from build123d import *

# Parameters (mm, degrees)
F1_DEPTH  = 6.35
F3_W      = 31.75
F3_H      = 6.35
F4_DEPTH  = 82.55
F6_DEPTH  = 6.35
F9_W      = 3.175
F9_H      = 12.7
F10_DEPTH = 222.25


with BuildPart() as f1:
    # F0 (on Front) → F1 (new body)
    with BuildSketch(Plane.XZ):
        Polygon((-41.275, 64.447084), (-41.275, 104.775), (-111.125, 104.775), align=None)
        Polygon((0, 104.775), (-41.275, 104.775), (-41.275, 64.447084), (-41.275, -53.975), (0, -53.975), align=None)
    extrude(amount=-F1_DEPTH)

    # F2: F1 across plane


with BuildPart() as f1_1:
    add(f1.part)
    add(f1.part.mirror(Plane.YZ))

    # F3 (on Front) → F4 (join)
    with BuildSketch(Plane.XZ):
        with Locations((0, -50.8)):
            Rectangle(F3_W, F3_H)
    extrude(amount=F4_DEPTH)

    # F5 (on face) → F6 (join)
    with BuildSketch(Plane.YZ.offset(15.875)):
        Polygon((0, -22.225), (-25.4, -47.625), (0, -47.625), align=None)
    extrude(amount=-F6_DEPTH)

    # F7: F1 across plane


with BuildPart() as f1_2:
    add(f1_1.part)
    add(f1_1.part.mirror(Plane.YZ))

    # F9 (on offset) → F10 (cut)
    with BuildSketch(Plane.YZ.offset(111.125)):
        with Locations((1.5875, 98.425)):
            Rectangle(F9_W, F9_H)
    extrude(amount=-F10_DEPTH, mode=Mode.SUBTRACT)


solid = f1_2.part
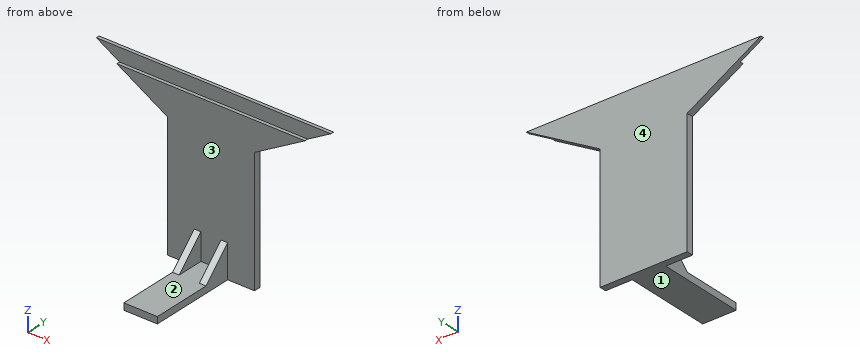
Geometry check sheet. Reference: the model listing, model coordinates, mm. Face numbers are marked on the shaded views. A direction names the side the tool comes from. Round coordinates to 2 decimals unless told otherwise and drop trailing zeros. Write each loop counter-clockwise with the first axis right and the second up, starting at its lowest first coordinate (ties: lowest second). Pieces come first, ordered by that corner, then holes.
Item 1: Material ranges on line 1 along Z through (x, y) = (-15, -55) (3 decimals); line 2 along Y through (x, z) = (-35, 33), recorded low to high.
Determined:
line 1: z = -53.975 to -47.625
line 2: y = 0 to 6.35
Item 2: Section check B-B (y = -17). Record the boundary of the cut face in (x, z) (3 decimals), plus the area to 3 significant figures.
Determined:
outline: (-15.875, -53.975) - (15.875, -53.975) - (15.875, -39.225) - (9.525, -39.225) - (9.525, -47.625) - (-9.525, -47.625) - (-9.525, -39.225) - (-15.875, -39.225) - close
area: 308 mm2
Item 3: Access from +Z, -Z, +X, -X, +Y, -Y to the whole of each face (thin tool, end or side, straight path). Record for the marked faces 3 and 4.
Determined:
face 3: +Z, -Y
face 4: +Z, -Z, +X, -X, +Y
Item 4: Go/stop test with flat-tipped pins: pin 1 Ø16 at (x, y) = (-6.5, -22.5) entering from +Z; pin 2 Ø14 at (x, z) = (-11.5, 100.5) entering from -Y (3 decimals); pin 3 Ø1.9 at (y, z) = (4, -9) entering from +X (3 decimals). Record where each tip stops, or that it passes through.
Determined:
pin 1: stops at z = -37.32
pin 2: stops at y = 3.175
pin 3: stops at x = 41.275
Item 5: Section check D-D (y = -70). Record the boundary of the cut face in (x, z) (3 decimals), plus the area to 3 significant figures.
Determined:
outline: (-15.875, -53.975) - (15.875, -53.975) - (15.875, -47.625) - (-15.875, -47.625) - close
area: 202 mm2
Item 6: Section check A-A (x = 5.5). Record the boundary of the cut face in (y, z) (3 decimals), plus the area to 3 significant figures.
Determined:
outline: (-82.55, -53.975) - (6.35, -53.975) - (6.35, 104.775) - (3.175, 104.775) - (3.175, 92.075) - (0, 92.075) - (0, -47.625) - (-82.55, -47.625) - close
area: 1,490 mm2
Item 7: Section check C-C (z = 57). Record the boundary of the cut face in (x, y) (3 decimals).
Determined:
outline: (-41.275, 0) - (41.275, 0) - (41.275, 6.35) - (-41.275, 6.35) - close
Item 8: Mould release check, pull along X, two halves, no side actions. Record for the marked faces 1 and 2: +X half, -X half, draft (parallel to the pull), parting line (faces both ways), or undercut.
Determined:
face 1: draft
face 2: undercut
